from build123d import *

# Parameters (mm, degrees)
SKETCH1_W           = 140
SKETCH1_H           = 160
BOSS_EXTRUDE1_DEPTH = 3
SKETCH2_W           = 120
SKETCH2_H           = 120
SKETCH2_W_2         = 117
SKETCH2_H_2         = 117
BOSS_EXTRUDE2_DEPTH = 70
SKETCH4_W           = 120
SKETCH4_H           = 120
BOSS_EXTRUDE4_DEPTH = 3
SKETCH5_R           = 2.1
SKETCH5_W           = 39.9
SKETCH5_H           = 19.71
CUT_EXTRUDE2_DEPTH  = 3
SKETCH6_W           = 18.298163042
SKETCH6_H           = 17.309993256
CUT_EXTRUDE3_DEPTH  = 3
CUT_EXTRUDE8_DEPTH  = 5
SKETCH15_W          = 259.021634325
SKETCH15_H          = 180.269434884
BOSS_EXTRUDE5_DEPTH = 3
SKETCH18_R          = 1.6
CUT_EXTRUDE9_DEPTH  = 10
SKETCH19_W          = 12
SKETCH19_H          = 4.5
SKETCH19_H_2        = 8.4
SKETCH19_W_2        = 10.084057066
SKETCH19_H_3        = 7.362028533
CUT_EXTRUDE11_DEPTH = 5


with BuildPart() as part:
    # Sketch1 → Boss-Extrude1 (new body)
    with BuildSketch(Plane(origin=(0, 0, 0), x_dir=(1, 0, 0), z_dir=(0, 1, 0))):
        Rectangle(SKETCH1_W, SKETCH1_H)
    extrude(amount=BOSS_EXTRUDE1_DEPTH)

    # Sketch2 → Boss-Extrude2 (add)
    with BuildSketch(Plane(origin=(0, 3, 0), x_dir=(1, 0, 0), z_dir=(0, 1, 0))):
        Rectangle(SKETCH2_W, SKETCH2_H)
        Rectangle(SKETCH2_W_2, SKETCH2_H_2, mode=Mode.SUBTRACT)
    extrude(amount=BOSS_EXTRUDE2_DEPTH)

    # Sketch4 → Boss-Extrude4 (add)
    with BuildSketch(Plane(origin=(0, 73, 0), x_dir=(1, 0, 0), z_dir=(0, 1, 0))):
        Rectangle(SKETCH4_W, SKETCH4_H)
    extrude(amount=BOSS_EXTRUDE4_DEPTH)

    # Sketch5 → Cut-Extrude2 (cut)
    with BuildSketch(Plane(origin=(0, 76, 0), x_dir=(1, 0, 0), z_dir=(0, 1, 0))):
        with Locations(Location((34.39, -4.925, 0), (0, 0, 270))):
            Circle(SKETCH5_R)
        with Locations(Location((34.39, 4.925, 0), (0, 0, 270))):
            Circle(SKETCH5_R)
        with Locations(Location((-15.03, -4.925, 0), (0, 0, 270))):
            Circle(SKETCH5_R)
        with Locations(Location((-15.03, 4.925, 0), (0, 0, 270))):
            Circle(SKETCH5_R)
        with Locations((9.68, 0)):
            Rectangle(SKETCH5_W, SKETCH5_H)
    extrude(amount=-CUT_EXTRUDE2_DEPTH, mode=Mode.SUBTRACT)

    # Sketch6 → Cut-Extrude3 (cut)
    with BuildSketch(Plane(origin=(0, 76, 0), x_dir=(1, 0, 0), z_dir=(0, 1, 0))):
        Rectangle(SKETCH6_W, SKETCH6_H)
    extrude(amount=-CUT_EXTRUDE3_DEPTH, mode=Mode.SUBTRACT)

    # Sketch13 → Cut-Extrude8 (cut)
    with BuildSketch(Plane(origin=(0, 76, 0), x_dir=(1, 0, 0), z_dir=(0, 1, 0))):
        with BuildLine():
            ThreePointArc((-3.792582359, 49.728765052), (-53.491503795, -1.722579942), (-0.349490011, -49.609426409))
            ThreePointArc((-0.349490011, -49.609426409), (5.82592347, -42.51288634), (-1.270616599, -36.337472859))
            ThreePointArc((-1.270616599, -36.337472859), (-40.195607742, -1.261740085), (-3.792582359, 36.42488497))
            ThreePointArc((-3.792582359, 36.42488497), (2.859357682, 43.076825011), (-3.792582359, 49.728765052))
        make_face()
    extrude(amount=-CUT_EXTRUDE8_DEPTH, mode=Mode.SUBTRACT)

    # Sketch15 → Boss-Extrude5 (add)
    with BuildSketch(Plane(origin=(0, 3, 0), x_dir=(1, 0, 0), z_dir=(0, 1, 0))):
        with Locations((-39.510817163, -10.134717442)):
            Rectangle(SKETCH15_W, SKETCH15_H)
    extrude(amount=-BOSS_EXTRUDE5_DEPTH)

    # Sketch18 → Cut-Extrude9 (cut)
    with BuildSketch(Plane(origin=(0, 3, 0), x_dir=(1, 0, 0), z_dir=(0, 1, 0))):
        with Locations(Location((-55.452, -27.227420358, 0), (0, 0, 270))):
            Circle(SKETCH18_R)
        with Locations(Location((-55.452, 32.208579642, 0), (0, 0, 270))):
            Circle(SKETCH18_R)
        with Locations(Location((4.746, 32.208579642, 0), (0, 0, 270))):
            Circle(SKETCH18_R)
        with Locations(Location((4.746, -27.227420358, 0), (0, 0, 270))):
            Circle(SKETCH18_R)
    extrude(amount=-CUT_EXTRUDE9_DEPTH, mode=Mode.SUBTRACT)

    # Sketch19 → Cut-Extrude11 (cut)
    with BuildSketch(Plane.ZY.offset(60)):
        with Locations((12.367420358, 33)):
            Rectangle(SKETCH19_W, SKETCH19_H)
        with Locations((-11.259414931, 37.2)):
            Rectangle(SKETCH19_W, SKETCH19_H_2)
        with Locations((-28.606781654, 36.742945388)):
            Rectangle(SKETCH19_W_2, SKETCH19_H_3)
    extrude(amount=-CUT_EXTRUDE11_DEPTH, mode=Mode.SUBTRACT)


solid = part.part
Check sheet for the modelled part. Datum: model origin and axes. Units: mm. A direction names the side the tool comes from. Round coordinates to 2 decimals unless told otherwise and drop trailing zeros. Loops run counter-clockwise (first coordinate to the right, second up) from the corner with the lowest first, then second, coordinate; pieces in that order, holes last. Notation, with made-up numbers: (66.5, -24) -> (72.5, -24) arc R27 cw to (72.5, 1) -> close; hole circle Ø5 at (-13, -25). An arc over 180 degrees is marked (long way). Put each result on its own line as item: value. Start each with the question number.
1. Section check A-A (y = 66.5). Enter the section's corners in (x, z).
2. Section check B-B (z = 0). Enter the section's corners in (x, y), plus the area to 3 significant figures.
3. Draft check along Z on faces 6 (the face through (-70, 3, 9)), 7 (the face through (-1, 73, -14)), 8 (the face through (-1, 39, -60)). Enter one of: +Z half, -Z half, draft (parallel to the pull), parting line (faces both ways), or undercut.
4. Section check D-D (z = 53.5). Enter the section's corners in (x, y).
5. Access from +Z, -Z, +X, -X, +Y, -Y to the whole of each face (thin tool, end or side, straight path). Record for faces 1 (the face through (-1, 39, 60)), 2 (the face through (-58.5, 38, 1)), 3 (the face through (-60, 39, 1)), 4 (the face through (60, 39, 1)), 5 (the face through (2.858, 74.521, -42.931)).
6. Gauge pin test, flat ends, axial feed: pin 1 (6 mm diameter, centred on y = 56.5, z = 48, fed in from +X); pin 2 (1.5 mm diameter, centred on x = 13, y = 75, fed in from -Z); pin 3 (1.6 mm diameter, centred on x = -59.5, y = 32.5, fed in from +Z). Record the tip position at first contact, or that the pin passes through.
7. Scan lines: probe 1 along X at (y, z) = (29, -30); probe 2 along Z at (x, y) = (34, 75). Record each from-to range of solid material in increasing order.
8. Section check C-C (x = 24). Enter the section's corners in (y, z) (3 decimals).
Findings:
1. outline: (-60, -60) -> (60, -60) -> (60, 60) -> (-60, 60) -> close; hole (-58.5, -58.5) -> (58.5, -58.5) -> (58.5, 58.5) -> (-58.5, 58.5) -> close
2. outline: (-169.02, 0) -> (90, 0) -> (90, 3) -> (60, 3) -> (60, 76) -> (29.63, 76) -> (29.63, 73) -> (58.5, 73) -> (58.5, 3) -> (-58.5, 3) -> (-58.5, 73) -> (-53.52, 73) -> (-53.52, 76) -> (-60, 76) -> (-60, 3) -> (-169.02, 3) -> close; (-40.22, 73) -> (-10.27, 73) -> (-10.27, 76) -> (-40.22, 76) -> close
2. area: 1,190 mm^2
3. face 6: draft
3. face 7: undercut
3. face 8: -Z half
4. outline: (-169.02, 0) -> (90, 0) -> (90, 3) -> (60, 3) -> (60, 76) -> (-60, 76) -> (-60, 3) -> (-169.02, 3) -> close; hole (-58.5, 3) -> (58.5, 3) -> (58.5, 73) -> (-58.5, 73) -> close
5. face 1: +Z, +X, -X, +Y
5. face 2: none
5. face 3: +Z, -Z, -X, +Y
5. face 4: +Z, -Z, +X, +Y
5. face 5: +Y
6. pin 1: stops at x = 60
6. pin 2: stops at z = -60
6. pin 3: stops at z = 60
7. probe 1: x = -60 to -58.5, 58.5 to 60
7. probe 2: z = -60 to -6.99, -2.86 to 2.86, 6.99 to 60
8. outline: (0, -80) -> (3, -80) -> (3, -60) -> (76, -60) -> (76, -9.855) -> (73, -9.855) -> (73, -58.5) -> (3, -58.5) -> (3, 58.5) -> (73, 58.5) -> (73, 9.855) -> (76, 9.855) -> (76, 60) -> (3, 60) -> (3, 100.269) -> (0, 100.269) -> close
